Autodesk Fusion 360 part; units mm, degrees
sketch "Sketch1" plane through (0, 0, 0) normal (0, 1, 0) x (1, 0, 0)
  line L0 (0, 0) -> (-36, 0)
  line L1 (-36, 0) -> (-36, 20)
  circle A0 centre (0, -82) radius 9
  circle A1 centre (0, -82) radius 18
  line L2 (0, 0) -> (36, 0)
  line L3 (82, 0) -> (118, 0)
  line L4 (118, 0) -> (118, 10)
  line L5 (118, 10) -> (78.9666, 10)
  line L6 (49.0334, 10) -> (43.0334, 10)
  line L7 (43.0334, 10) -> (43.0334, 20)
  line L8 (-36, 20) -> (44.4041, 20)
  arc A2 (44.4041, 20) -> (90.1534, 10) centre (64, 0) ccw
  arc A3 (49.0334, 10) -> (78.9666, 10) centre (64, 0) ccw
  line L9 (12.0259, -95.3932) -> (84.3038, -19.281)
  line L10 (-36, 0) -> (-17.5996, -85.7754)
  line L11 (0, 0) -> (5, 0)
  line L12 (5, 0) -> (5, -64.7084)
  line L13 (0, 0) -> (-5, 0)
  line L14 (-5, 0) -> (-5, -64.7084)
  dimension "d1" = 36
  dimension "d2" = 20
  dimension "d4" = 82
  dimension "d5" = 18
  dimension "d6" = 36
  dimension "d7" = 64
  dimension "d8" = 36
  dimension "d9" = 56
  dimension "d12" = 54
  dimension "d13" = 10
  dimension "d14" = 6
  dimension "d15" = 10
  dimension "d22" = 5
  dimension "d23" = 64.7084
  dimension "d24" = 5
extrude "Extrude1" add sketch "Sketch1" along normal mid plane 72 contours L0 L1 L2 L7 L8 A2 L11 L13 | L3 L6 L7 A2 A3 | L3 L4 L5 A2 | L3 L5 A2 A3 makes body 1
extrude "Extrude2" add sketch "Sketch1" along normal mid plane 54 separate body contours A1 L9 | A1 L9 makes body 2
extrude "Extrude3" add sketch "Sketch1" along normal mid plane 54 contours L0 A1 L2 L11 L12 L13 L14 bodies 2
extrude "Extrude4" add sketch "Sketch1" along normal mid plane 10 contours L0 A1 L10 L14 bodies 1 2
extrude "Extrude5" add sketch "Sketch1" along normal mid plane 10 contours A1 L2 A2 L9 L12 bodies 1
sketch "Sketch4" plane through (0, 0, 0) normal (0, 0, 1) x (1, 0, 0)
  line L0 (0, 0) -> (18, 0)
  line L1 (108, -10) -> (128, -10)
  line L2 (128, -10) -> (128, 10)
  line L3 (128, 10) -> (108, 10)
  line L4 (108, 10) -> (108, -10)
  line L5 (108, -10) -> (128, 10) construction
  line L6 (128, -10) -> (108, 10) construction
  point P0 (118, 0)
  dimension "d31" = 18
  dimension "d40" = 20
  dimension "d41" = 20
hole "Hole1" at (18.0126, -18.0267, 0) direction (0, 0, -1) diameter 12 depth 30 tip angle 118 bodies 1
hole "Hole2" at (17.8831, 17.9931, 0) direction (0, 0, -1) diameter 12 depth 30 tip angle 118 bodies 1
extrude "Extrude6" cut sketch "Sketch4" against normal blind 20 bodies 1
Can you work these out from the model? Positions are in its coordinate system, mm. A direction names the side the tool comes from. Give positions to 0.01 mm unless a question says otherwise; leave off trailing zeros. Loops run counter-clockwise (first coordinate to the right, second up) from the corner with the lowest first, then second, coordinate; pieces in that order, holes last. Notation, with made-up numbers: M 44,89.25 L 86,89.25 A10 cw 86,104.25 Z; hole C -17.5,-34.75 d6. An arc over 180 degrees is marked long. Use one line per item in the form item = value. Start each with the question number.
(1) I'm going to push flat-ended pins straight in: P1, Ø4, axis at y = 11.5, z = 54, coming from the -X side; P2, Ø2, axis at x = -13.5, z = 6, coming from the -Y side; P3, Ø1, axis at x = 79, y = 7, coming from the -Z side; P4, Ø14, axis at x = 18.01, y = -18.03, coming from the -Z side. Where does each tip first touch, or does it pass through?
(2) I want a section at C-C, the plane x = 0. Write out the boundary of the cut face in (y, z), and give its area (3 significant figures).
(3) I want a section at B-B, the plane z = 82. Write out the boundary of the cut face in (x, y).
(4) On a 3-axis mill with a long thin cutter (end or side, diameter ignored), from which of +Z, -Z, +X, -X, +Y, -Y can I reach the whole of each face in a straight line? I mean faces 4 (the cylindrical face through (16.21, -23.75, -10.14)), 5 (the flat face through (105, -1, 0)), 6 (the flat face through (43.033, -1, -15)), 7 (the flat face through (113, -10, -5)). Say none if no direction works.
(5) I want a section at D-D, the plane x = 56. Write out the boundary of the cut face in (y, z).
(6) I want a section at A-A, the plane y = 14.5. Write out the boundary of the cut face in (x, z), and give its area (3 significant figures).
(7) Please list where these lines run through material, in increasing order: line 1 (Z direction, x = 0, y = -8); line 2 (Y direction, x = 12, z = 13.5); line 3 (X direction, y = -5.5, z = 15.5).
(8) Thinking about a two-plate mould opening in Y: for faces 1 (the flat face through (113, 10, -5)), 2 (the flat face through (-36, -1, -10)), 3 (the flat face through (23, -36, -2)), which applies, released by +Y, released by -Y, zero draft, split by the parting line, or undercut?
Worked out:
q1.P1 = -5
q1.P2 = -5
q1.P3 = -10
q1.P4 = -20
q2.outline = M -36,-20 L 36,-20 L 36,0 L 27,0 L 27,73 L -27,73 L -27,0 L -36,0 Z; M -27,91 L 27,91 L 27,100 L -27,100 Z
q2.area = 5,870 mm²
q3.outline = M -18.41,-5 L -18,-5 L -18,-27 L -9,-27 L -9,27 L -18,27 L -18,5 L -18.41,5 Z; M 9,-27 L 18,-27 L 18,-5 L 24.74,-5 L 24.74,5 L 18,5 L 18,27 L 9,27 Z
q4.face_4 = -Z
q4.face_5 = +Z, +X, +Y, -Y
q4.face_6 = -Z, +X, +Y, -Y
q4.face_7 = +Z, -Z, +X
q5.outline = M -36,16.12 L 36,16.12 L 36,26.83 L 5,26.83 L 5,49.09 L -5,49.09 L -5,26.83 L -36,26.83 Z
q6.outline = M -36,-20 L 13,-20 L 13,0 L 5,0 L 5,64.71 A18 ccw long -5,64.71 L -5,0 L -36,0 Z; M 22.76,-20 L 43.03,-20 L 43.03,-10 L 49.03,-10 A18 cw long 78.97,-10 L 118,-10 L 118,0 L 92,0 A28 ccw 36,0 L 22.76,0 Z; hole C 0,82 d18
q6.area = 3,920 mm²
q7.line_1 = -20 to 73, 91 to 100
q7.line_2 = -5 to 5
q7.line_3 = -5 to 5, 40.68 to 54.85, 73.15 to 87.32
q8.face_1 = undercut
q8.face_2 = zero draft
q8.face_3 = released by -Y
